Geometry check sheet. Reference: the model listing, model coordinates, mm. A direction names the side the tool comes from. Give positions to 0.01 mm unless a question says otherwise; leave off trailing zeros. Write each loop counter-clockwise with the first axis right and the second up, starting at its lowest first coordinate (ties: lowest second). Pieces come first, ordered by that corner, then holes.
(1) Cross-section at A-A (x = 0). Count the separate pieces of the cut face and the enclosed holes in it, and give its area (3 significant figures).
(2) Thickness scan on line 1 along Z through (x, y) = (-20, 4.25); line 2 along Z through (x, y) = (19, 6.5); line 3 along X through (y, z) = (2.75, 103.17). Record the ranges inside material, lowest first.
(3) Cross-section at D-D (x = 26). Record the boundary of the cut face in (y, z).
(4) Cross-section at B-B (z = 70). Record the boundary of the cut face in (x, y).
(5) Tool access check on faces 1 (the flat face through (-21.15, 5, 70)), 2 (the flat face through (-18.7, 5.1, 51.4)), 3 (the cylindrical face through (5.39, 6.3, 23.55)). Record the directions out of +Z, -Z, +X, -X, +Y, -Y that give a thin tool (end or side, any length) a straight path to the whole face; none if there is none.
(6) Mould release check, pull along X, two halves, no side actions. Record for faces 4 (the flat face through (-18.6, 5.1, 88.7)), 5 (the flat face through (7, 3, 25)), 6 (the cylindrical face through (1.22, 4.93, -34.98)): +X half, -X half, draft (parallel to the pull), parting line (faces both ways), or undercut.
(7) Depth check by flat-ended pin: P1, Ø1.3, axis at x = -15.5, y = 5.5, coming from the -Z side; P2, Ø4, axis at x = -14, y = 5, coming from the +Z side; P3, Ø4.5, axis at x = 15.494, z = 85.494, coming from the +Y side. Enter the tip coordinate at first touch or a pass-through.
(8) Cross-section at C-C (z = 25). Record the boundary of the cut face in (x, y) (3 decimals).
```python
from build123d import *

# Parameters (mm, degrees)
SKETCH1_R                                      = 35
BOSS_EXTRUDE1_DEPTH                            = 10
SKETCH3_R                                      = 3.75
CUT_EXTRUDE1_DEPTH                             = 10
SKETCH4_R                                      = 5
BOSS_EXTRUDE2_DEPTH                            = 10
CBORE_FOR_4_SOCKET_HEAD_CAP_SCREW1_D           = 3.2639
CBORE_FOR_4_SOCKET_HEAD_CAP_SCREW1_CBORE_D     = 5.55752
CBORE_FOR_4_SOCKET_HEAD_CAP_SCREW1_CBORE_DEPTH = 2.8448
CHAMFER1_SIZE                                  = 5
SKETCH9_R                                      = 11.43
CUT_EXTRUDE5_DEPTH                             = 2.54
FILLET2_R                                      = 15
FILLET3_R                                      = 5
SKETCH16_R                                     = 5
CUT_EXTRUDE9_DEPTH                             = 115.130403048
CUT_EXTRUDE9_DRAFT                             = 10
SKETCH12_R                                     = 2.5
CUT_EXTRUDE6_DEPTH                             = 115.130403048
CBORE_FOR_M4_SHCS1_OUTLINE_R                   = 4.003586442
CBORE_FOR_M4_SHCS1_OUTLINE_R_2                 = 2.5
CBORE_FOR_M4_SHCS1_DEPTH                       = 4
SKETCH22_W                                     = 80
SKETCH22_H                                     = 20
CUT_EXTRUDE11_DEPTH                            = 3
SKETCH23_R                                     = 1.825
CUT_EXTRUDE12_DEPTH                            = 7
CHAMFER2_SIZE                                  = 0.5


# Read off the part's stored shape, not the designer's step: CBORE for M4 SHCS1
with BuildPart() as part:
    # Sketch1 → Boss-Extrude1 (new body)
    with BuildSketch(Plane(origin=(0, 0, 0), x_dir=(1, 0, 0), z_dir=(0, 1, 0))):
        with Locations(Location((0, 0, 0), (0, 0, 270))):
            Circle(SKETCH1_R)
    extrude(amount=BOSS_EXTRUDE1_DEPTH)

    # Sketch3 → Cut-Extrude1 (cut)
    with BuildSketch(Plane(origin=(0, 10, 0), x_dir=(1, 0, 0), z_dir=(0, 1, 0))):
        with Locations(Location((-17.67766953, 17.67766953, 0), (0, 0, 270))):
            Circle(SKETCH3_R)
        with Locations(Location((17.67766953, 17.67766953, 0), (0, 0, 270))):
            Circle(SKETCH3_R)
        with Locations(Location((17.67766953, -17.67766953, 0), (0, 0, 270))):
            Circle(SKETCH3_R)
        with Locations(Location((-17.67766953, -17.67766953, 0), (0, 0, 270))):
            Circle(SKETCH3_R)
    extrude(amount=-CUT_EXTRUDE1_DEPTH, mode=Mode.SUBTRACT)

    # Sketch4 → Boss-Extrude2 (add)
    with BuildSketch(Plane(origin=(0, 10, 0), x_dir=(1, 0, 0), z_dir=(0, 1, 0))):
        Polygon((-15, -48.85), (-21.15, -48.85), (-21.15, -91.15), (-7.5, -91.15), (-7.5, -108.17), (7.5, -108.17), (7.5, -91.15), (21.15, -91.15), (21.15, -48.85), (15, -48.85), (15, -31.622776602), (-15, -31.622776602), align=None)
        with Locations(Location((0, -70, 0), (0, 0, 270))):
            Circle(SKETCH4_R, mode=Mode.SUBTRACT)
    extrude(amount=-BOSS_EXTRUDE2_DEPTH)

    # CBORE for #4 Socket Head Cap Screw1 (through all)
    with Locations(Plane(origin=(-15.494, 10, 54.506), x_dir=(0, 0, 1), z_dir=(0, 1, 0))):
        with Locations((0, 0), (0, 30.988), (30.988, 30.988), (30.988, 0)):
            CounterBoreHole(CBORE_FOR_4_SOCKET_HEAD_CAP_SCREW1_D / 2, CBORE_FOR_4_SOCKET_HEAD_CAP_SCREW1_CBORE_D / 2, CBORE_FOR_4_SOCKET_HEAD_CAP_SCREW1_CBORE_DEPTH)

    # Chamfer1
    chamfer1_edges = [part.edges().sort_by_distance(p)[0] for p in [
        (-21.15, 5, 91.15),
        (-21.15, 5, 48.85),
        (21.15, 5, 48.85),
        (21.15, 5, 91.15),
    ]]
    chamfer(chamfer1_edges, length=CHAMFER1_SIZE)

    # Sketch9 → Cut-Extrude5 (cut)
    with BuildSketch(Plane(origin=(0, 0, 0), x_dir=(-1, 0, 0), z_dir=(0, -1, 0))):
        with Locations(Location((0, -70, 0), (0, 0, 90))):
            Circle(SKETCH9_R)
    extrude(amount=-CUT_EXTRUDE5_DEPTH, mode=Mode.SUBTRACT)

    # Fillet2
    fillet2_edges = [part.edges().sort_by_distance(p)[0] for p in [
        (-15, 5, 31.622776602),
        (15, 5, 31.622776602),
    ]]
    fillet(fillet2_edges, radius=FILLET2_R)

    # Fillet3
    fillet3_edges = [part.edges().sort_by_distance(p)[0] for p in [
        (7.5, 5, 91.15),
        (-7.5, 5, 91.15),
    ]]
    fillet(fillet3_edges, radius=FILLET3_R)


with BuildPart() as cut_extrude9_tool:
    # Sketch16 → Cut-Extrude9 (with draft: the straight prism first)
    with BuildSketch(Plane(origin=(0, 0, 0), x_dir=(-1, 0, 0), z_dir=(0, -1, 0))):
        Circle(SKETCH16_R)
    extrude(amount=-CUT_EXTRUDE9_DEPTH)
    # Cut-Extrude9: the draft: its side faces are tilted about the plane it starts from
    cut_extrude9_sides = [cut_extrude9_tool.faces().sort_by_distance(p)[0] for p in [
        (5, 57.565201524, 0),
    ]]
    draft(cut_extrude9_sides, Plane(origin=(0, 0, 0), x_dir=(-1, 0, 0), z_dir=(0, -1, 0)), CUT_EXTRUDE9_DRAFT)


with BuildPart() as part_1:
    add(part.part)

    # Cut-Extrude9: cut by cut_extrude9_tool
    add(cut_extrude9_tool.part, mode=Mode.SUBTRACT)

    # Sketch12 → Cut-Extrude6 (cut, through all)
    with BuildSketch(Plane(origin=(0, 0, 0), x_dir=(-1, 0, 0), z_dir=(0, -1, 0))):
        with Locations(Location((0, -36.67, 0), (0, 0, 90))):
            Circle(SKETCH12_R)
        with Locations(Location((0, -103.17, 0), (0, 0, 90))):
            Circle(SKETCH12_R)
    extrude(amount=-CUT_EXTRUDE6_DEPTH, mode=Mode.SUBTRACT)

    # CBORE for M4 SHCS1 outline → CBORE for M4 SHCS1 (cut)
    with BuildSketch(Plane(origin=(0, 0, 0), x_dir=(1, 0, 0), z_dir=(0, 1, 0))):
        with Locations((0, -36.67)):
            Circle(CBORE_FOR_M4_SHCS1_OUTLINE_R)
        with Locations((0, -36.67)):
            Circle(CBORE_FOR_M4_SHCS1_OUTLINE_R_2, mode=Mode.SUBTRACT)
    extrude(amount=CBORE_FOR_M4_SHCS1_DEPTH, mode=Mode.SUBTRACT)

    # Sketch22 → Cut-Extrude11 (cut)
    with BuildSketch(Plane(origin=(0, 10, 0), x_dir=(1, 0, 0), z_dir=(0, 1, 0))):
        Rectangle(SKETCH22_W, SKETCH22_H)
    extrude(amount=-CUT_EXTRUDE11_DEPTH, mode=Mode.SUBTRACT)

    # Sketch23 → Cut-Extrude12 (cut)
    with BuildSketch(Plane(origin=(0, 10, 0), x_dir=(1, 0, 0), z_dir=(0, 1, 0))):
        with Locations(Location((-6.5, 25, 0), (0, 0, 270))):
            Circle(SKETCH23_R)
        with Locations(Location((6.5, 25, 0), (0, 0, 270))):
            Circle(SKETCH23_R)
        with Locations(Location((6.5, -25, 0), (0, 0, 270))):
            Circle(SKETCH23_R)
        with Locations(Location((-6.5, -25, 0), (0, 0, 270))):
            Circle(SKETCH23_R)
    extrude(amount=-CUT_EXTRUDE12_DEPTH, mode=Mode.SUBTRACT)

    # Chamfer2
    chamfer2_edges = [part_1.edges().sort_by_distance(p)[0] for p in [
        (-6.5, 10, -26.825),
        (6.5, 10, -26.825),
        (6.5, 10, 23.175),
        (-6.5, 10, 23.175),
    ]]
    chamfer(chamfer2_edges, length=CHAMFER2_SIZE)


solid = part_1.part
```
Reply:
1. separate pieces: 5
1. enclosed holes: 0
1. area: 1,050 mm2
2. line 1: z = -28.72 to -20.62, -14.73 to 14.73, 20.62 to 28.82, 52.7 to 87.3
2. line 2: z = -29.39 to -21.19, -14.17 to 14.17, 21.19 to 29.8, 51.7 to 88.3
2. line 3: x = -7.5 to -2.5, 2.5 to 7.5
3. outline: (0, -23.43) - (10, -23.43) - (10, -10) - (7, -10) - (7, 10) - (10, 10) - (10, 23.43) - (0, 23.43) - close
4. outline: (-21.15, 0) - (-11.43, 0) - (-11.43, 2.54) - (-5, 2.54) - (-5, 10) - (-21.15, 10) - close; (5, 2.54) - (11.43, 2.54) - (11.43, 0) - (21.15, 0) - (21.15, 10) - (5, 10) - close
5. face 1: +Z, -X, +Y, -Y
5. face 2: -X, +Y, -Y
5. face 3: +Y
6. face 4: -X half
6. face 5: undercut
6. face 6: parting line
7. P1: stops at z = -31.69
7. P2: stops at z = 91.18
7. P3: stops at y = 7.16
8. outline: (-24.495, 0) - (24.495, 0) - (24.495, 10) - (8.825, 10) - (8.325, 9.5) - (8.325, 3) - (4.675, 3) - (4.675, 9.5) - (4.175, 10) - (-4.175, 10) - (-4.675, 9.5) - (-4.675, 3) - (-8.325, 3) - (-8.325, 9.5) - (-8.825, 10) - (-24.495, 10) - close
